Check sheet for the modelled part. Datum: model origin and axes. Units: mm. Coordinates: 2 decimals unless noted, no trailing zeros. Write each loop counter-clockwise with the first axis right and the second up, starting at its lowest first coordinate (ties: lowest second). Pieces come first, ordered by that corner, then holes. Notation, with made-up numbers: M 15.5,43.5 L 57.5,43.5 A15 ccw 57.5,69.5 Z; hole C 88,55 d4. An arc over 180 degrees is marked long. Answer as CSV lines item,"result".
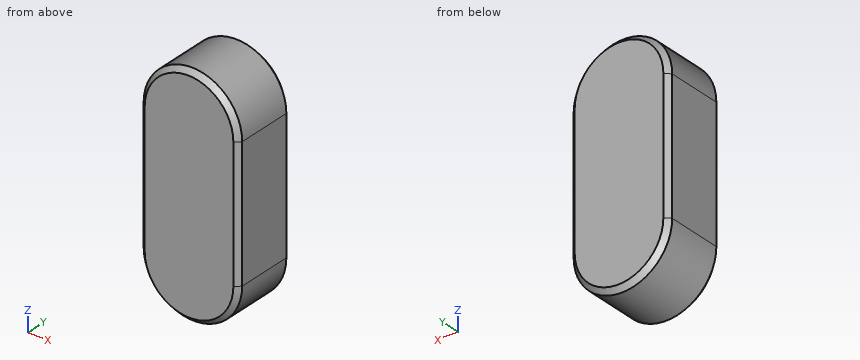
from build123d import *

# Parameters (mm, degrees)
BOSS_EXTRUDE1_DEPTH = 8
CHAMFER1_SIZE       = 0.6


with BuildPart() as part:
    # Sketch1 → Boss-Extrude1 (new body)
    with BuildSketch(Plane(origin=(0, 0, 0), x_dir=(1, 0, 0), z_dir=(0, 1, 0))):
        with BuildLine():
            Line((6, 0), (6, 16))
            ThreePointArc((6, 16), (0, 22), (-6, 16))
            Line((-6, 16), (-6, 0))
            ThreePointArc((-6, 0), (0, -6), (6, 0))
        make_face()
    extrude(amount=BOSS_EXTRUDE1_DEPTH)

    # Chamfer1
    chamfer1_edges = [part.edges().sort_by_distance(p)[0] for p in [
        (0, 8, -22),
        (-6, 8, -8),
        (0, 8, 6),
        (-6, 0, -8),
        (0, 0, -22),
        (6, 0, -8),
        (0, 0, 6),
        (6, 8, -8),
    ]]
    chamfer(chamfer1_edges, length=CHAMFER1_SIZE)


solid = part.part
1) Thickness scan on line 1 along X through (y, z) = (6.25, 0.25); line 2 along X through (y, z) = (3.5, -18.5); line 3 along Z through (x, y) = (3.5, 4.5). Record the ranges inside material, lowest first.
Answer key:
line 1,"x = -5.99 to 5.99"
line 2,"x = -5.45 to 5.45"
line 3,"z = -20.87 to 4.87"
2) Section check A-A, the plane y = 3.75. Record the boundary of the cut face in (x, z), plus the area to 3 significant figures.
Answer key:
outline,"M -6,-16 A6 ccw 6,-16 L 6,0 A6 ccw -6,0 Z"
area,"305 mm2"
3) Depth check by flat-ended pin: P1, Ø1, axis at x = -2.5, y = 3, coming from the +Z side. Enter the tip coordinate at first touch or a pass-through.
Answer key:
P1,"stops at z = 5.66"
